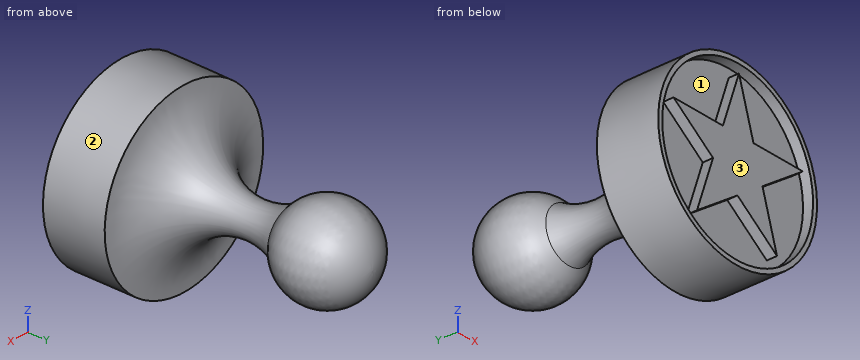
Autodesk Fusion 360 part; units mm, degrees
sketch "草图1" plane through (0, 0, 0) normal (1, 0, 0) x (0, 0, -1)
  line L0 (-26, 1) -> (-26, 18)
  arc A0 (-26, 18) -> (-7.7417, 49.3746) centre (-26, 39) ccw
  arc A1 (-0.1986, 73.1451) -> (-7.7417, 49.3746) centre (0, 60) ccw
  line L1 (-26, 1) -> (-26, 0)
  line L2 (-26, 0) -> (0, 0)
  line L3 (0, 0) -> (-0.1986, 73.1451)
revolve "旋转1" add sketch "草图1" angle 360 about axis through (0, 0, 0) along (0, 1, 0.0027)
sketch "草图2" plane through (0, 0, 0) normal (0, 1, 0) x (1, 0, 0)
  circle A0 centre (0, 0) radius 24.6982
extrude "拉伸1" cut sketch "草图2" along normal blind 3
sketch "草图3" plane through (0, 0, 0) normal (0, 1, 0) x (1, 0, 0)
  line L0 (-21.0825, -7.217) -> (21.2981, -6.5533)
  line L1 (-13.3786, 17.8204) -> (0.349, -22.2808)
  line L2 (12.814, 18.2307) -> (0.349, -22.2808)
  line L3 (-21.0825, -7.217) -> (12.814, 18.2307)
  line L4 (-13.3786, 17.8204) -> (21.2981, -6.5533)
extrude "拉伸2" add sketch "草图3" along normal blind 3
Read the model definition and answer for the solid it produces. Units are mm, in the model's axes. Face numbers are marked on the shaded views. Coordinates: 2 decimals unless noted, no trailing zeros. Answer as a JSON object with one key per item and string values.
Q1. Consider line 1 (X direction, y = 1, z = 0); line 2 (Y direction, x = -23.5, z = 6); line 3 (Y direction, x = 17, z = -8.5). Determine where each line is inside the solid, lowest interval first. Write a range as [from, to].
The answers:
{"line 1": "x = [-26, -24.7], [-11.47, 11.97], [24.7, 26]", "line 2": "y = [3, 18.12]", "line 3": "y = [3, 19.25]"}
Q2. Determine the mould class of the marked faces 1, 2 and 3 for opening direction X: pulls with the +X half, pulls with the -X half, needs draft (parallel to the pull), parting line crosses it, or undercut.
The answers:
{"face 1": "undercut", "face 2": "parting line crosses it", "face 3": "needs draft"}
Q3. Flat-ended cylindrical pins translate along their axes: pin 1 Ø8 at (y, z) = (52, -12.5) entering from -X; pin 2 Ø2 at (x, z) = (-17, -8) entering from -Y; pin 3 Ø3 at (x, z) = (-1, 11.5) entering from +Y. Find the tip coordinate at first contact, or state that the pin passes through.
The answers:
{"pin 1": "stops at x = -6.97", "pin 2": "stops at y = 3", "pin 3": "stops at y = 68.48"}
